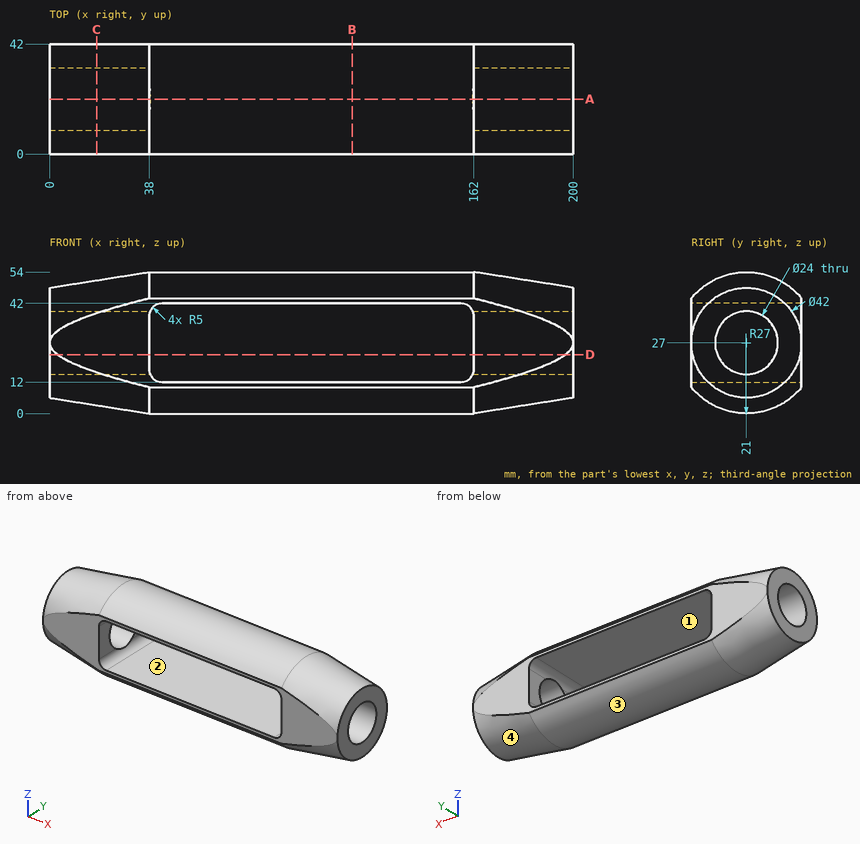
Print and shaded views of the part. All mm, measured from the part's lowest x, y and z. Coordinates: 2 decimals unless noted, no trailing zeros. Order: outer loops, then holes, each group sorted by start corner. A loop starts at its lowest first (then second) coordinate and runs counter-clockwise, first axis right, second up. Notation, with made-up numbers: M -37,-25.5 L 18,-25.5 A17 cw 18,6.5 Z; hole C 31.5,-32 d3. An arc over 180 degrees is marked long. Write each question's results on one line, items separated by ' | '. Start each with the question number.
Q1. Cut at D-D (z = 22.5). Count the separate pieces of the cut face and the enclosed holes in it, then the cut area to 3 significant figures.
Q2. Cut at A-A (y = 21). List the corners of the cut face in (x, z), then the cut area to 3 significant figures.
Q3. Drill centre lines: probe 1 along Y at (x, z) = (11.5, 27); probe 2 along X at (y, z) = (38.5, 23); probe 3 along Z at (x, y) = (107, 4). Where is each one in solid material? Low to high. Write a range as from..to.
Q4. Cut at B-B (x = 115.5). List the corners of the cut face in (y, z).
Q5. Pull direction X, two halves, no side cores. Call the marked faces 1, 2, 3 and 4: +X half, -X half, draft (parallel to the pull), parting line (faces both ways), or undercut.
Q6. Flat gauge pins, fed straight in: P1, Ø8, axis at x = 60.5, y = 14, coming from the +Z side; P2, Ø10, axis at x = 28, z = 48, coming from the +Y side. Where does each tip first touch, or does it go through?
Q7. Cut at C-C (x = 18). List the corners of the cut face in (y, z), then the cut area to 3 significant figures.
Found:
1) separate pieces: 4 | enclosed holes: 0 | area: 1,500 mm²
2) outline: M 0,6 L 38,0 L 162,0 L 200,6 L 200,15 L 161.58,15 A5 cw 157,12 L 43,12 A5 cw 38.42,15 L 0,15 Z; M 0,39 L 38.42,39 A5 cw 43,42 L 157,42 A5 cw 161.58,39 L 200,39 L 200,48 L 162,54 L 38,54 L 0,48 Z | area: 4,820 mm²
3) probe 1: 0..9, 33..42 | probe 2: 0..38, 162..200 | probe 3: 6.02..12, 42..47.98
4) outline: M 0,10.03 A27 ccw 42,10.03 L 42,12 L 0,12 Z; M 0,42 L 42,42 L 42,43.97 A27 ccw 0,43.97 Z
5) face 1: undercut | face 2: undercut | face 3: draft | face 4: +X half
6) P1: z = 53.83 | P2: y = 40.88
7) outline: M 0,15.71 A23.84 ccw 42,15.71 L 42,38.29 A23.84 ccw 0,38.29 Z; hole C 21,27 d24 | area: 1,250 mm²
